from build123d import *

# Parameters (mm, degrees)
SKETCH1_W                    = 70.78
SKETCH1_H                    = 128.4
BULK_DEPTH                   = 2.5
MOUNT_HOLE_NW_DEPTH          = 141.506579561
MOUNT_HOLES_NE_SE_COUNT      = 2
MOUNT_HOLES_NE_SE_PITCH      = 55.88
MOUNT_HOLES_NE_SE_COUNT_DIR2 = 2
MOUNT_HOLES_NE_SE_PITCH_DIR2 = 122.4
MOUNT_HOLE_SW_DEPTH          = 141.506579561
ALIGNMENT_HOLE_D             = 3
DRILL_HOLES_AT_2_COUNT       = 2
DRILL_HOLES_AT_2_PITCH       = 74
DRILL_HOLES_AT_3_COUNT       = 2
DRILL_HOLES_AT_3_PITCH       = 95.72313409
DRILL_HOLES_AT_4_COUNT       = 2
DRILL_HOLES_AT_4_PITCH       = 60.72
SKETCH9_W                    = 10
SKETCH9_H                    = 12.5
USB_DEPTH                    = 141.506579561
MCXX_DEPTH                   = 141.506579561
SKETCH12_R                   = 4.5
SELECTOR_1_DEPTH             = 141.506579561
COPY_SELECTOR_COUNT          = 3
COPY_SELECTOR_PITCH          = 12
MMCX_2_DEPTH                 = 141.506579561
SKETCH25_R                   = 1.5
SKETCH25_W                   = 9.5
SKETCH25_H                   = 11
BARREL_JACK_DEPTH            = 141.506579561


with BuildPart() as part:
    # Sketch1 → Bulk (new body)
    with BuildSketch(Plane.XY.offset(2.5)):
        with Locations((27.94, 61.2)):
            Rectangle(SKETCH1_W, SKETCH1_H)
    extrude(amount=-BULK_DEPTH)

    # Sketch2 → Mount hole NW (cut, through all)
    with BuildSketch(Plane.XY.offset(2.5)):
        with BuildLine():
            Line((2.445403852, 124.05), (-2.445403852, 124.05))
            ThreePointArc((-2.445403852, 124.05), (-2.95, 122.4), (-2.445403852, 120.75))
            Line((-2.445403852, 120.75), (2.445403852, 120.75))
            ThreePointArc((2.445403852, 120.75), (2.95, 122.4), (2.445403852, 124.05))
        make_face()
    mount_hole_nw = extrude(amount=-MOUNT_HOLE_NW_DEPTH, mode=Mode.SUBTRACT)

    # Mount holes NE SE: Mount hole NW 2 × 2, 1 skipped
    with Locations(*[(i * MOUNT_HOLES_NE_SE_PITCH, -j * MOUNT_HOLES_NE_SE_PITCH_DIR2, 0) for i in range(MOUNT_HOLES_NE_SE_COUNT) for j in range(MOUNT_HOLES_NE_SE_COUNT_DIR2) if (i, j) not in ((0, 0), (0, 1))]):
        add(mount_hole_nw, mode=Mode.SUBTRACT)

    # Sketch3 → Mount hole SW (cut, through all)
    with BuildSketch(Plane.XY.offset(2.5)):
        with BuildLine():
            Line((7.525403852, 1.65), (2.634596148, 1.65))
            ThreePointArc((2.634596148, 1.65), (2.13, 0), (2.634596148, -1.65))
            Line((2.634596148, -1.65), (7.525403852, -1.65))
            ThreePointArc((7.525403852, -1.65), (8.03, 0), (7.525403852, 1.65))
        make_face()
    extrude(amount=-MOUNT_HOLE_SW_DEPTH, mode=Mode.SUBTRACT)

    # Alignment hole (through all)
    with Locations(Plane.XY.offset(2.5)):
        with Locations((-3.95, 119.1)):
            Hole(ALIGNMENT_HOLE_D / 2)

    # Sketch7 → Drill holes (revolve, cut)
    with BuildSketch(Plane(origin=(-2.42, 24.2, 2.5), x_dir=(0, -1, 0), z_dir=(1, 0, 0))):
        Polygon((0, 0), (0, 2.5), (1.35, 2.5), (1.35, 1.5), (2.5, 0.35), (2.5, 0), align=None)
    drill_holes = revolve(axis=Axis((-2.42, 24.2, 8.85), (0, 0, -1)), mode=Mode.SUBTRACT)

    # Drill holes at 2: Drill holes ×2
    with Locations(*[(0, i * DRILL_HOLES_AT_2_PITCH, 0) for i in range(1, DRILL_HOLES_AT_2_COUNT)]):
        add(drill_holes, mode=Mode.SUBTRACT)

    # Drill holes at 3: Drill holes ×2
    with Locations(*[Vector(0.6343294186643587, 0.7730628620086059, 0) * (i * DRILL_HOLES_AT_3_PITCH) for i in range(1, DRILL_HOLES_AT_3_COUNT)]):
        add(drill_holes, mode=Mode.SUBTRACT)

    # Drill holes at 4: Drill holes ×2
    with Locations(*[(i * DRILL_HOLES_AT_4_PITCH, 0, 0) for i in range(1, DRILL_HOLES_AT_4_COUNT)]):
        add(drill_holes, mode=Mode.SUBTRACT)

    # Sketch9 → USB (cut, through all)
    with BuildSketch(Plane.XY.offset(2.5)):
        with Locations((6.61, 26.2)):
            Rectangle(SKETCH9_W, SKETCH9_H)
    extrude(amount=-USB_DEPTH, mode=Mode.SUBTRACT)

    # Sketch10 → MCXX (cut, through all)
    with BuildSketch(Plane.XY.offset(2.5)):
        Polygon((6.61, 49.2), (6.61, 37.2), (6.61, 33.2), (10.61, 33.2), (10.61, 37.2), (10.61, 49.2), align=None)
    extrude(amount=-MCXX_DEPTH, mode=Mode.SUBTRACT)

    # Sketch12 → Selector 1 (cut, through all)
    with BuildSketch(Plane.XY.offset(2.5)):
        with Locations((13.11, 53.2)):
            Circle(SKETCH12_R)
    selector_1 = extrude(amount=-SELECTOR_1_DEPTH, mode=Mode.SUBTRACT)

    # Copy selector: Selector 1 ×3
    with Locations(*[(0, i * COPY_SELECTOR_PITCH, 0) for i in range(1, COPY_SELECTOR_COUNT)]):
        add(selector_1, mode=Mode.SUBTRACT)

    # Sketch27 → MMCX 2 (cut, through all)
    with BuildSketch(Plane.XY.offset(2.5)):
        Polygon((6.61, 101.2), (6.61, 88.2), (6.61, 84.2), (10.61, 84.2), (10.61, 88.2), (10.61, 101.2), align=None)
    extrude(amount=-MMCX_2_DEPTH, mode=Mode.SUBTRACT)

    # Sketch25 → Barrel Jack (cut, through all)
    with BuildSketch(Plane.XY.offset(2.5)):
        with Locations((23.043898983, 22.557406324)):
            Circle(SKETCH25_R)
        with Locations((23.043898983, 7.257406324)):
            Circle(SKETCH25_R)
        with Locations((23.043898983, 15.057406324)):
            Rectangle(SKETCH25_W, SKETCH25_H)
    extrude(amount=-BARREL_JACK_DEPTH, mode=Mode.SUBTRACT)


solid = part.part
Verification items for the finished model (mm, model axes). Give positions to 0.01 mm unless a question says otherwise; leave off trailing zeros. Write each loop counter-clockwise with the first axis right and the second up, starting at its lowest first coordinate (ties: lowest second). Pieces come first, ordered by that corner, then holes. Notation, with made-up numbers: M 24.25,-20.75 L 59.25,-20.75 A21 cw 59.25,3.25 Z; hole C 28.5,42.25 d5. An arc over 180 degrees is marked long. Write item = value, one per line.
(1) Sectioned sample at B-B (y = 98.2). Record the cut outline in (x, z), then the cut area to 3 significant figures.
Found:
outline = M -7.45,0 L -3.77,0 L -3.77,1 L -4.92,2.15 L -4.92,2.5 L -7.45,2.5 Z; M -1.07,0 L 6.61,0 L 6.61,2.5 L 0.08,2.5 L 0.08,2.15 L -1.07,1 Z; M 10.61,0 L 56.95,0 L 56.95,1 L 55.8,2.15 L 55.8,2.5 L 10.61,2.5 Z; M 59.65,0 L 63.33,0 L 63.33,2.5 L 60.8,2.5 L 60.8,2.15 L 59.65,1 Z
area = 149 mm2
(2) Material ranges on line 1 (Y direction, x = 6.5, z = 0.25); line 2 (X direction, y = 24.2, z = 0.85); line 3 (X direction, y = 98.2, z = 0.75), recorded low to high.
Found:
line_1 = -3 to -1.65, 1.65 to 19.95, 32.45 to 125.4
line_2 = -7.45 to -3.77, -1.07 to 1.61, 11.61 to 56.95, 59.65 to 63.33
line_3 = -7.45 to -3.77, -1.07 to 6.61, 10.61 to 56.95, 59.65 to 63.33
(3) Sectioned sample at A-A (y = 14). Record the cut outline in (x, z), then the cut area to 3 significant figures.
Found:
outline = M -7.45,0 L 18.29,0 L 18.29,2.5 L -7.45,2.5 Z; M 27.79,0 L 63.33,0 L 63.33,2.5 L 27.79,2.5 Z
area = 153 mm2
(4) Go/stop test with flat-tipped pins: pin 1 Ø14.5 at (x, y) = (13.11, 77.2) entering from +Z; pin 2 Ø3 at (x, y) = (-2.42, 24.2) entering from +Z. Record where each tip stops, or that it passes through.
Found:
pin_1 = 2.5
pin_2 = 1.15
(5) Sectioned sample at D-D (y = 77.2). Record the cut outline in (x, z), then the cut area to 3 significant figures.
Found:
outline = M -7.45,0 L 8.61,0 L 8.61,2.5 L -7.45,2.5 Z; M 17.61,0 L 63.33,0 L 63.33,2.5 L 17.61,2.5 Z
area = 154 mm2
(6) Sectioned sample at C-C (x = 13.11). Record the cut outline in (y, z), then the cut area to 4 significant figures.
Found:
outline = M -3,0 L 48.7,0 L 48.7,2.5 L -3,2.5 Z; M 57.7,0 L 60.7,0 L 60.7,2.5 L 57.7,2.5 Z; M 69.7,0 L 72.7,0 L 72.7,2.5 L 69.7,2.5 Z; M 81.7,0 L 125.4,0 L 125.4,2.5 L 81.7,2.5 Z
area = 253.5 mm2
(7) Draft check along X on faces 1 (the face through (63.33, 60, 1)), 2 (the face through (0.02, 24.74, 2.33)). Enter one of: released by +X, released by -X, zero draft, split by the parting line, or undercut.
Found:
face_1 = released by +X
face_2 = undercut
